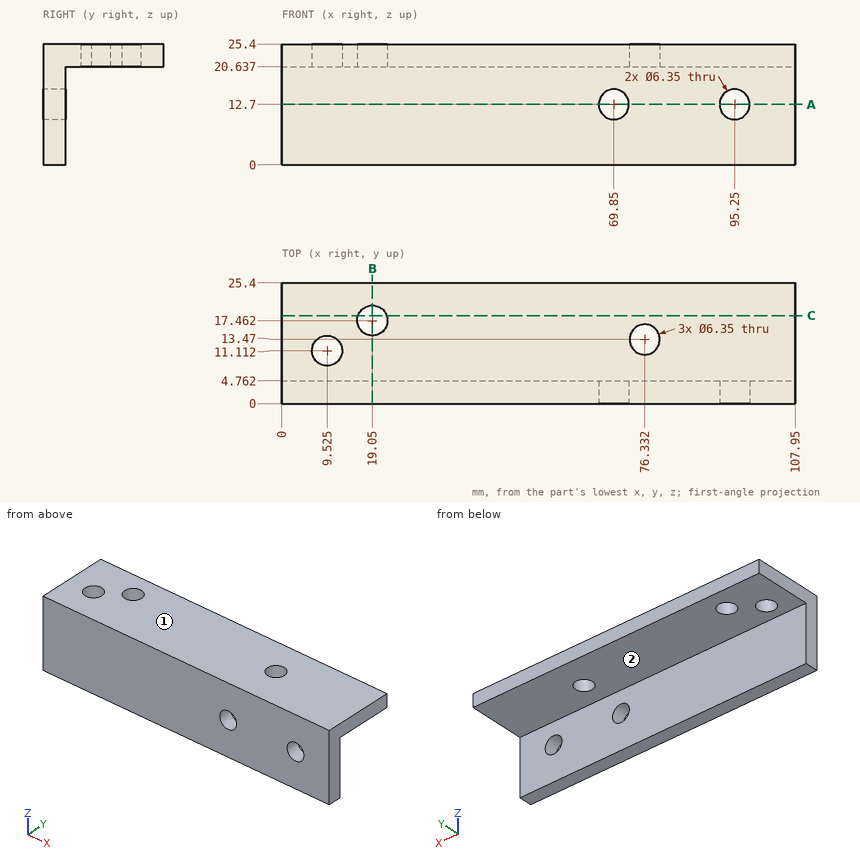
Source: three-view drawing plus pictorial views. Frame: mm from the lowest corner of the part. A direction names the side the tool comes from. Round coordinates to 2 decimals unless told otherwise and drop trailing zeros. Order: outer loops, then holes, each group sorted by start corner. A loop starts at its lowest first (then second) coordinate and runs counter-clockwise, first axis right, second up. Notation, with made-up numbers: (-28, 82) - (18, 82) arc R12 ccw to (18, 100) - close; hole circle Ø7 at (-18.5, -0.5). An arc over 180 degrees is marked (long way). Answer in a Markdown table with one row per item.
Item 1: Line query: line 1 (Y direction, x = 48.5, z = 15); line 2 (Z direction, x = 54, y = 7.25). Output: solid intervals per line, ascending.
Model answer:
| item | result |
|---|---|
| line 1 | y = 0 to 4.76 |
| line 2 | z = 20.64 to 25.4 |
Item 2: Section query C-C (y = 18.5). Return the cut outline in (x, z).
Model answer:
| item | result |
|---|---|
| outline | (0, 20.64) - (16.05, 20.64) - (16.05, 25.4) - (0, 25.4) - close; (22.05, 20.64) - (107.95, 20.64) - (107.95, 25.4) - (22.05, 25.4) - close |
Item 3: Section query B-B (x = 19.05). Return the cut outline in (y, z).
Model answer:
| item | result |
|---|---|
| outline | (0, 0) - (4.76, 0) - (4.76, 20.64) - (14.29, 20.64) - (14.29, 25.4) - (0, 25.4) - close; (20.64, 20.64) - (25.4, 20.64) - (25.4, 25.4) - (20.64, 25.4) - close |
Item 4: Reachability of the marked faces 1 and 2 from +Z, -Z, +X, -X, +Y, -Y: full face, straight path, thin tool, end or side. Return the list, or none.
Model answer:
| item | result |
|---|---|
| face 1 | +Z, +X, -X, +Y, -Y |
| face 2 | -Z, +X, -X, +Y |
Item 5: Pin query (flat end, axial travel): pin 1 (7.5 mm diameter, centred on x = 69.85, z = 12.7, fed in from +Y); pin 2 (8 mm diameter, centred on x = 75.5, y = 19.5, fed in from -Z). Return the tip coordinate at first contact, or that it passes through.
Model answer:
| item | result |
|---|---|
| pin 1 | stops at y = 4.76 |
| pin 2 | stops at z = 20.64 |
Item 6: Section query A-A (z = 12.7). Give the number of separate pieces and of enclosed holes in the cut face.
Model answer:
| item | result |
|---|---|
| separate pieces | 3 |
| enclosed holes | 0 |
